```python
from build123d import *

# Parameters (mm, degrees)
SKETCH1_R               = 53.34
SKETCH1_R_2             = 50.8
BOSS_EXTRUDE1_DEPTH     = 812.8
CUT_EXTRUDE1_REACH      = 818.293
CUT_EXTRUDE1_END_RADIUS = 53.34
SKETCH2_W               = 152.4
SKETCH2_H               = 5.08
CIRPATTERN1_COUNT       = 4


with BuildPart() as part:
    # Sketch1 → Boss-Extrude1 (new body)
    with BuildSketch(Plane.XY):
        Circle(SKETCH1_R)
        Circle(SKETCH1_R_2, mode=Mode.SUBTRACT)
    extrude(amount=BOSS_EXTRUDE1_DEPTH)

    # Cut-Extrude1: up to this cylinder (the profile starts inside it)
    cut_extrude1_end = Plane(origin=(0, 0, 88.9), z_dir=(0, 0, -1)) * Cylinder(CUT_EXTRUDE1_END_RADIUS, 1744.266, mode=Mode.PRIVATE)
    # Sketch2 → Cut-Extrude1 (cut, up to the surface)
    with BuildSketch(Plane(origin=(0, 0, 0), x_dir=(0, 0, -1), z_dir=(1, 0, 0)), mode=Mode.PRIVATE) as cut_extrude1_sk1:
        with Locations((-88.9, 0)):
            Rectangle(SKETCH2_W, SKETCH2_H)
    cut_extrude1_tool1 = extrude(cut_extrude1_sk1.sketch, amount=-CUT_EXTRUDE1_REACH, mode=Mode.PRIVATE) & cut_extrude1_end
    cut_extrude1 = cut_extrude1_tool1.solids().sort_by_distance((0, 0, 88.9))[0]
    add(cut_extrude1, mode=Mode.SUBTRACT)

    # CirPattern1: Cut-Extrude1 ×4 about axis
    cirpattern1_axis = Axis((0, 0, 0), (0, 0, 1))
    for i in range(1, CIRPATTERN1_COUNT):
        add(cut_extrude1.rotate(cirpattern1_axis, i * 360 / CIRPATTERN1_COUNT), mode=Mode.SUBTRACT)


solid = part.part
```
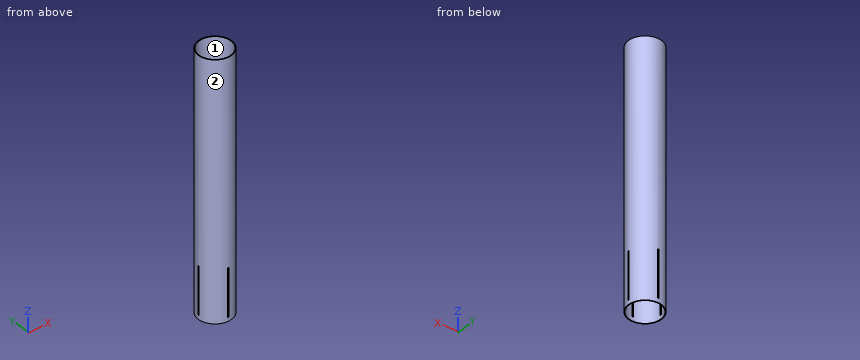
Build history of the part. All positions in model axes, mm. Face numbers are marked on the shaded views. Round coordinates to 2 decimals unless told otherwise and drop trailing zeros. Write each loop counter-clockwise with the first axis right and the second up, starting at its lowest first coordinate (ties: lowest second). Pieces come first, ordered by that corner, then holes. Notation, with made-up numbers: (8, 77) - (17, 77) arc R21 cw to (17, 101) - close; hole circle Ø1 at (-2, 11). An arc over 180 degrees is marked (long way). Write each question's results on one line, items separated by ' | '. Start each with the question number.
Item 1: Saw through at B-B (x = -35). Write the cut outline in (y, z).
Item 2: Drop flat-ended pins along their axis: P1, Ø5, axis at x = -33.5, z = 411, coming from the -Y side; P2, Ø8, axis at x = 41, z = 166, coming from the -Y side; P3, Ø0.8, axis at x = -51.5, y = 0, coming from the -Z side; P4, Ø12, axis at y = -30.5, z = 445.5, coming from the +X side. Give the stop position or say it passes through.
Item 3: Mould opens along Y. For the marked faces 1 and 2 say: pulls with the +Y half, pulls with the -Y half, needs draft (parallel to the pull), parting line crosses it, or undercut.
Item 4: Saw through at C-C (z = 235.5). Write the cut outline in (x, y).
Item 5: Saw through at A-A (y = 26). Write the cut outline in (x, z), and give its area (3 significant figures).
Item 6: Wall check: L1, parallel to Y at x = -1, z = 375.5; L2, parallel to X at y = 0, z = 379.5; L3, parallel to Y at x = 17, z = 754.5. Give the ranges that are in metal, low to high. Write a range as [from, to].
Results are:
1) outline: (-40.25, 0) - (-36.82, 0) - (-36.82, 812.8) - (-40.25, 812.8) - close; (36.82, 0) - (40.25, 0) - (40.25, 812.8) - (36.82, 812.8) - close
2) P1: stops at y = -43.41 | P2: stops at y = -38.42 | P3: stops at z = 0 | P4: stops at x = 47.38
3) face 1: undercut | face 2: parting line crosses it
4) outline: circle Ø106.68 at (0, 0); hole circle Ø101.6 at (0, 0)
5) outline: (-46.57, 0) - (-43.64, 0) - (-43.64, 812.8) - (-46.57, 812.8) - close; (43.64, 0) - (46.57, 0) - (46.57, 812.8) - (43.64, 812.8) - close | area: 4,770 mm²
6) L1: y = [-53.33, -50.79], [50.79, 53.33] | L2: x = [-53.34, -50.8], [50.8, 53.34] | L3: y = [-50.56, -47.87], [47.87, 50.56]
